```python
from build123d import *

# Parameters (mm, degrees)
SKETCH1_W                    = 25
SKETCH1_H                    = 15
BASE_FLANGE1_DEPTH           = 3.175
EDGE_FLANGE1_STRIP_W         = 18.7
EDGE_FLANGE1_STRIP_H         = 3.175
EDGE_FLANGE1_STRIP_CUT_DEPTH = 15
EDGE_FLANGE1_DEPTH           = 15
EDGE_FLANGE2_STRIP_W         = 18.7
EDGE_FLANGE2_STRIP_H         = 3.175
EDGE_FLANGE2_STRIP_CUT_DEPTH = 15
EDGE_FLANGE2_DEPTH           = 15
SKETCH12_W                   = 15
SKETCH12_H                   = 3.175
BOSS_EXTRUDE1_DEPTH          = 45
SKETCH15_R                   = 2.54
CUT_EXTRUDE2_DEPTH           = 74.371128518
SKETCH19_W                   = 15
SKETCH19_H                   = 3.175
BOSS_EXTRUDE2_DEPTH          = 10
SKETCH21_R                   = 2.54
CUT_EXTRUDE3_DEPTH           = 75.668136611
FILLET2_R                    = 3
FILLET3_R                    = 10


# Sheet-metal steps are written as plain solids
with BuildPart() as part:
    # Sketch1 → Base-Flange1 (new body)
    with BuildSketch(Plane.XY):
        Rectangle(SKETCH1_W, SKETCH1_H)
    extrude(amount=-BASE_FLANGE1_DEPTH)

    # Edge-Flange1 strip (across the edge) → Edge-Flange1 strip cut (cut)
    with BuildSketch(Plane(origin=(12.5, 7.5, -3.175), x_dir=(-1, 0, 0), z_dir=(0, -1, 0))):
        with Locations((-6.35, -1.5875)):
            Rectangle(EDGE_FLANGE1_STRIP_W, EDGE_FLANGE1_STRIP_H)
    extrude(amount=EDGE_FLANGE1_STRIP_CUT_DEPTH, mode=Mode.SUBTRACT)

    # Edge-Flange1 section (across the edge) → Edge-Flange1 (add)
    with BuildSketch(Plane(origin=(12.5, 7.5, -3.175), x_dir=(-1, 0, 0), z_dir=(0, -1, 0))):
        with BuildLine():
            Line((-3.175, 3), (-3.175, 25.475))
            Line((-3.175, 25.475), (0, 25.475))
            Line((0, 25.475), (0, 3))
            ThreePointArc((0, 3), (0.878679656, 0.878679656), (3, 0))
            Line((3, 0), (3, -3.175))
            ThreePointArc((3, -3.175), (-1.366384374, -1.366384374), (-3.175, 3))
        make_face()
    extrude(amount=EDGE_FLANGE1_DEPTH)

    # Edge-Flange2 strip (across the edge) → Edge-Flange2 strip cut (cut)
    with BuildSketch(Plane(origin=(15.675, -7.5, -28.65), x_dir=(0, 0, 1), z_dir=(0, 1, 0))):
        with Locations((-6.35, -1.5875)):
            Rectangle(EDGE_FLANGE2_STRIP_W, EDGE_FLANGE2_STRIP_H)
    extrude(amount=EDGE_FLANGE2_STRIP_CUT_DEPTH, mode=Mode.SUBTRACT)

    # Edge-Flange2 section (across the edge) → Edge-Flange2 (add)
    with BuildSketch(Plane(origin=(15.675, -7.5, -28.65), x_dir=(0, 0, 1), z_dir=(0, 1, 0))):
        with BuildLine():
            Line((-3.175, 3), (-3.175, 26.825))
            Line((-3.175, 26.825), (0, 26.825))
            Line((0, 26.825), (0, 3))
            ThreePointArc((0, 3), (0.878679656, 0.878679656), (3, 0))
            Line((3, 0), (3, -3.175))
            ThreePointArc((3, -3.175), (-1.366384374, -1.366384374), (-3.175, 3))
        make_face()
    extrude(amount=EDGE_FLANGE2_DEPTH)

    # Sketch12 → Boss-Extrude1 (add)
    with BuildSketch(Plane(origin=(0, 7.5, 0), x_dir=(1, 0, 0), z_dir=(0, 1, 0))):
        with Locations((-5, 1.5875)):
            Rectangle(SKETCH12_W, SKETCH12_H)
    extrude(amount=BOSS_EXTRUDE1_DEPTH)

    # Sketch15 → Cut-Extrude2 (cut, through all)
    with BuildSketch(Plane(origin=(0, 0, -3.175), x_dir=(-1, 0, 0), z_dir=(0, 0, -1))):
        with Locations((5, 47.42)):
            Circle(SKETCH15_R)
    extrude(amount=-CUT_EXTRUDE2_DEPTH, mode=Mode.SUBTRACT)

    # Sketch19 → Boss-Extrude2 (add)
    with BuildSketch(Plane(origin=(0, 7.5, 0), x_dir=(1, 0, 0), z_dir=(0, 1, 0))):
        with Locations((35, 30.2375)):
            Rectangle(SKETCH19_W, SKETCH19_H)
    extrude(amount=BOSS_EXTRUDE2_DEPTH)

    # Sketch21 → Cut-Extrude3 (cut, through all)
    with BuildSketch(Plane(origin=(0, 0, -31.825), x_dir=(-1, 0, 0), z_dir=(0, 0, -1))):
        with Locations((-35, 12.42)):
            Circle(SKETCH21_R)
    extrude(amount=-CUT_EXTRUDE3_DEPTH, mode=Mode.SUBTRACT)

    # Fillet2
    fillet2_edges = [part.edges().sort_by_distance(p)[0] for p in [
        (42.5, 17.5, -30.2375),
        (27.5, 17.5, -30.2375),
        (-12.5, 52.5, -1.5875),
        (2.5, 52.5, -1.5875),
    ]]
    fillet(fillet2_edges, radius=FILLET2_R)

    # Fillet3
    fillet3_edges = [part.edges().sort_by_distance(p)[0] for p in [
        (42.5, -7.5, -30.2375),
        (-12.5, -7.5, -1.5875),
    ]]
    fillet(fillet3_edges, radius=FILLET3_R)


solid = part.part
```
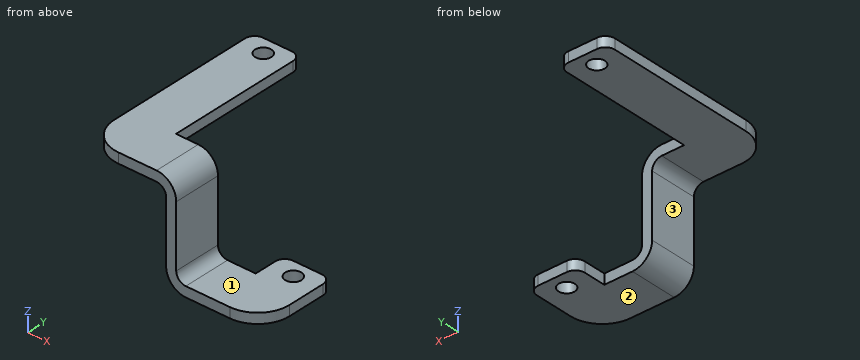
Work out the finished part from the listing and answer in its coordinate system (mm). Face numbers are marked on the shaded views. A direction names the side the tool comes from. Round coordinates to 2 decimals unless told otherwise and drop trailing zeros. Loops run counter-clockwise (first coordinate to the right, second up) from the corner with the lowest first, then second, coordinate; pieces in that order, holes last. Notation, with made-up numbers: (-12, -11) -> (9, -11) arc R21 cw to (9, 0) -> close; hole circle Ø7 at (24.25, 26.25). An arc over 180 degrees is marked (long way). Write each question's results on one line, items separated by ' | '. Start each with the question number.
1. Section A-A (y = 12.42) is taken. Determine the outline of the cut face in (x, z) (3 decimals).
2. A tool of negligible diameter and unlimited length cuts with its end or side. For the marked faces 1, 2 and 3, from which of +Z, -Z, +X, -X, +Y, -Y can it reach the whole face along a straight path? Write none if from no direction.
3. Given pin 1 Ø2.5 at (x, z) = (34, -30) entering from +Y; pin 2 Ø2.5 at (y, z) = (12.5, -30) entering from -X; pin 3 Ø16.5 at (y, z) = (1.5, -20.5) entering from -X, each flat-ended and moving along its own axis, determine where each tip first touches the part or whether it passes through.
4. Section C-C (x = 35) is taken. Determine the outline of the cut face in (y, z) (3 decimals), plus the area to 3 significant figures.
5. Section D-D (z = -15) is taken. Determine the outline of the cut face in (x, y) (3 decimals), plus the area to 3 significant figures.
6. Section B-B (y = 47.42) is taken. Determine the outline of the cut face in (x, z) (3 decimals).
7. Find the intervals of material crossed by probe 1 along Z at (x, y) = (-9, 27) (3 decimals); probe 2 along Z at (x, y) = (23, 3.5) (3 decimals); probe 3 along X at (y, z) = (12, -31), in increasing order. Write a range as from..to.
Evaluation:
1) outline: (-12.5, -3.175) -> (2.5, -3.175) -> (2.5, 0) -> (-12.5, 0) -> close; (27.5, -31.825) -> (32.46, -31.825) -> (32.46, -28.65) -> (27.5, -28.65) -> close; (37.54, -31.825) -> (42.5, -31.825) -> (42.5, -28.65) -> (37.54, -28.65) -> close
2) face 1: +Z, +X, +Y, -Y | face 2: -Z, +X, -X, +Y, -Y | face 3: -Z, -X, +Y, -Y
3) pin 1: stops at y = 17.5 | pin 2: stops at x = 27.5 | pin 3: stops at x = 12.5
4) outline: (-7.182, -31.825) -> (9.88, -31.825) -> (9.88, -28.65) -> (-7.182, -28.65) -> close; (14.96, -31.825) -> (17.5, -31.825) -> (17.5, -28.65) -> (14.96, -28.65) -> close | area: 62.2 mm2
5) outline: (12.5, -7.5) -> (15.675, -7.5) -> (15.675, 7.5) -> (12.5, 7.5) -> close | area: 47.6 mm2
6) outline: (-12.5, -3.175) -> (-7.54, -3.175) -> (-7.54, 0) -> (-12.5, 0) -> close; (-2.46, -3.175) -> (2.5, -3.175) -> (2.5, 0) -> (-2.46, 0) -> close
7) probe 1: z = -3.175..0 | probe 2: z = -31.825..-28.65 | probe 3: x = 27.5..32.49, 37.51..42.5
